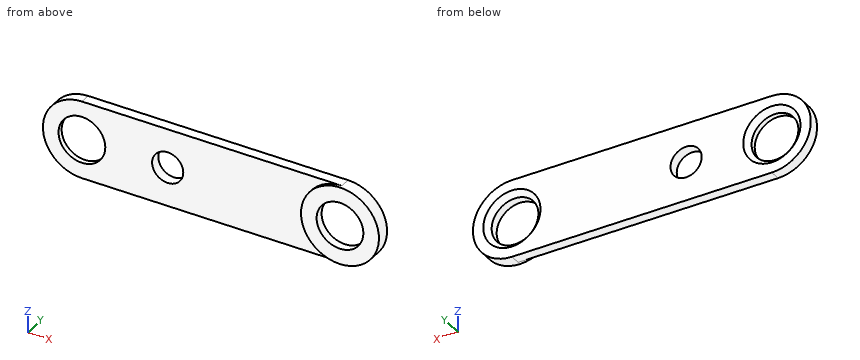
Autodesk Fusion 360 part; units mm, degrees
sketch "Sketch1" plane through (0, 0, 0) normal (0, 1, 0) x (1, 0, 0)
  line L0 (10.6191, -31.3581) -> (94.7803, -31.3581) construction
  line L1 (17.4831, -11.9367) -> (17.4831, -43.2834) construction
  line L2 (67.4831, -11.9367) -> (67.4831, -43.2834) construction
  circle A0 centre (17.4831, -31.3581) radius 7.5
  circle A1 centre (67.4831, -31.3581) radius 7.5
  line L3 (10.4242, -23.8581) -> (76.5455, -23.8581) construction
  line L4 (7.5967, -38.8581) -> (83.3606, -38.8581) construction
  line L5 (17.4831, -23.8581) -> (67.4831, -23.8581)
  line L6 (17.4831, -38.8581) -> (67.4831, -38.8581)
  circle A2 centre (67.4831, -31.3581) radius 4.5
  circle A3 centre (17.4831, -31.3581) radius 4.5
  line L7 (33.9831, -16.495) -> (33.9831, -43.6658) construction
  circle A4 centre (33.9831, -31.3581) radius 3
  dimension "d1" = 50
  dimension "d2" = 15
  dimension "d3" = 15
  dimension "d4" = 9
  dimension "d5" = 9
  dimension "d9" = 16.5
  dimension "d10" = 6
extrude "Extrude1" add sketch "Sketch1" along normal blind 2
chamfer "Chamfer1" distance 1 angle 45 2 edges at (13.2876, 2, 29.7308) (63.2876, 2, 29.7308)
sketch "Sketch2" plane through (0, 0, 0) normal (0, -1, 0) x (1, 0, 0)
  circle A0 centre (33.9831, 31.3581) radius 3
  circle A1 centre (17.4831, 31.3581) radius 4.5
  circle A2 centre (67.4831, 31.3581) radius 4.5
  arc A3 (17.4831, 38.8581) -> (17.4831, 23.8581) centre (17.4831, 31.3581) ccw
  line L0 (17.4831, 23.8581) -> (67.4831, 23.8581)
  arc A4 (67.4831, 23.8581) -> (67.4831, 38.8581) centre (67.4831, 31.3581) ccw
  line L1 (67.4831, 38.8581) -> (17.4831, 38.8581)
  circle A5 centre (67.4831, 31.3581) radius 7.5
  circle A6 centre (67.4831, 31.3581) radius 4.5
extrude "Extrude2" add sketch "Sketch2" along normal blind 0.6 contours A4 A5
The model under review builds one solid part; all positions refer to its coordinate system, in mm. Coordinates: 2 decimals unless noted, no trailing zeros. Order: outer loops, then holes, each group sorted by start corner. A loop starts at its lowest first (then second) coordinate and runs counter-clockwise, first axis right, second up. Notation, with made-up numbers: (17.5, 1.25) -> (28.5, 1.25) arc R22 ccw to (28.5, 14.25) -> close; hole circle Ø4 at (50.25, 13). An arc over 180 degrees is marked (long way). Answer in a Markdown table with one row per item.
(1) Insertion check: pin 1 (1.5 mm diameter, centred on y = 0, z = 29, fed in from -X); pin 2 (1 mm diameter, centred on y = 0.5, z = 30.5, fed in from -X); pin 3 (2 mm diameter, centred on x = 28, z = 35.5, fed in from -Y). Each pin has a flat end and moves straight along its axis. Give the tip position at first contact, or say it passes through.
Answers:
| item | result |
|---|---|
| pin 1 | x = 10.16 |
| pin 2 | x = 9.99 |
| pin 3 | y = 0 |
(2) Consider section D-D (z = 25). Write out the cut boundary in (x, y).
Answers:
| item | result |
|---|---|
| outline | (13.51, 0) -> (63.51, 0) -> (63.51, -0.6) -> (71.46, -0.6) -> (71.46, 2) -> (13.51, 2) -> close |
(3) Consider section A-A (z = 32.5). State how many separate pieces and enclosed holes the cut face has, plus the area to 3 significant figures.
Answers:
| item | result |
|---|---|
| separate pieces | 4 |
| enclosed holes | 0 |
| area | 85.3 mm² |
(4) Wall thickness on line 1 along X through (y, z) = (0.2, 33.5); line 2 along X through (y, z) = (0.5, 27.75); line 3 along X through (y, z) = (1.3, 34.5): over which ranges is each line inside the solid? List them lowest first.
Answers:
| item | result |
|---|---|
| line 1 | 10.3 to 13.53, 21.44 to 31.88, 36.08 to 63.53, 71.44 to 74.67 |
| line 2 | 10.91 to 14.79, 20.17 to 64.79, 70.17 to 74.06 |
| line 3 | 10.67 to 13.85, 21.11 to 63.85, 71.11 to 74.29 |
(5) Consider section B-B (x = 56). Write out the cut boundary in (y, z), plus the area to 3 significant figures.
Answers:
| item | result |
|---|---|
| outline | (0, 23.86) -> (2, 23.86) -> (2, 38.86) -> (0, 38.86) -> close |
| area | 30.0 mm² |
